Source: CAD feature listing. Evaluate the final solid. Frame: model axes, mm. Face numbers are marked on the shaded views. A direction names the side the tool comes from. Give positions to 0.01 mm unless a question says otherwise; leave off trailing zeros. Order: outer loops, then holes, each group sorted by start corner. A loop starts at its lowest first (then second) coordinate and runs counter-clockwise, first axis right, second up.
1) Section B-B, the plane z = 4.45. Return loops of the section in (x, y), plus the area to 3 significant figures.
2) Draft query along Z for the marked faces 1, 2, 3 and 4. Return one class per face: released by +Z, released by -Z, zero draft, split by the parting line, or undercut.
3) First-contact query: P1, Ø2, axis at y = 4, z = 1, coming from the -X side; P2, Ø1.5, axis at y = 4, z = 4.5, coming from the +X side; P3, Ø0.8, axis at y = 1.5, z = 3, coming from the +X side; P4, Ø0.8, axis at x = -0.5, z = 2.5, coming from the +Y side. Flat tips, straight axial feed; report the tip coordinate or a pass-through.
4) Section C-C, the plane z = 1. Return loops of the section in (x, y), plus the area to 3 significant figures.
5) Section A-A, the plane y = 0.5. Return loops of the section in (x, z).
6) Material intervals for line 1 (Z direction, x = 2, y = 0.3); line 2 (Z direction, x = 0.7, y = 4); line 3 (X direction, y = 1.75, z = 3.9), sorted ascending.
7) Section D-D, the plane x = 2.65. Return loops of the section in (y, z), plus the area to 3 significant figures.
8) Access query for the marked faces 5, 6 and 7. Directions: +Z, -Z, +X, -X, +Y, -Y. A direction counts if a zero-diameter tool reaches every point of the face in a straight line with its end or side. Return the directions, or none.
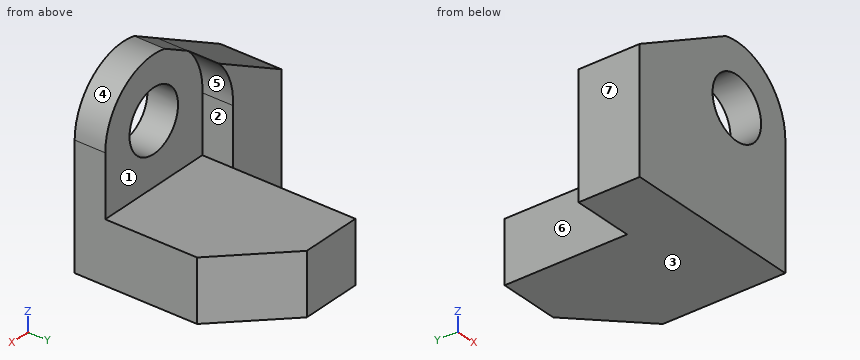
```python
from build123d import *

# Parameters (mm, degrees)
SKETCH1_R           = 1
BOSS_EXTRUDE1_DEPTH = 2
CUT_EXTRUDE1_DEPTH  = 1
SKETCH3_W           = 4
SKETCH3_H           = 2
BOSS_EXTRUDE2_DEPTH = 5
CHAMFER1_SIZE       = 2


with BuildPart() as part:
    # Sketch1 → Boss-Extrude1 (new body)
    with BuildSketch(Plane(origin=(0, 0, 0), x_dir=(1, 0, 0), z_dir=(0, 1, 0))):
        with BuildLine():
            Line((0, -4), (0, 0))
            Line((0, 0), (-2, 0))
            Line((-2, 0), (-2, -4))
            Line((-2, -4), (0.596081752, -5.424434468))
            ThreePointArc((0.596081752, -5.424434468), (0.15502893, -4.772063308), (0, -4))
        make_face()
        with BuildLine():
            Line((4, 0), (0, 0))
            Line((0, 0), (0, -4))
            ThreePointArc((0, -4), (0.15502893, -4.772063308), (0.596081752, -5.424434468))
            Line((0.596081752, -5.424434468), (1.552766589, -5.949354323))
            ThreePointArc((1.552766589, -5.949354323), (3.246100553, -5.56436358), (4, -4))
            Line((4, -4), (4, 0))
        make_face()
        with Locations((2, -4)):
            Circle(SKETCH1_R, mode=Mode.SUBTRACT)
    extrude(amount=BOSS_EXTRUDE1_DEPTH)

    # Sketch2 → Cut-Extrude1 (cut)
    with BuildSketch(Plane(origin=(0, 2, 0), x_dir=(1, 0, 0), z_dir=(0, 1, 0))):
        with BuildLine():
            Line((0, 0), (4, 0))
            Line((4, 0), (4, -4))
            ThreePointArc((4, -4), (1.935634166, -6.000972869), (0, -3.875221449))
            Line((0, -3.875221449), (0, 0))
        make_face()
    extrude(amount=-CUT_EXTRUDE1_DEPTH, mode=Mode.SUBTRACT)

    # Sketch3 → Boss-Extrude2 (add)
    with BuildSketch(Plane(origin=(0, 1, 0), x_dir=(1, 0, 0), z_dir=(0, 1, 0))):
        with Locations((2, -1)):
            Rectangle(SKETCH3_W, SKETCH3_H)
    extrude(amount=BOSS_EXTRUDE2_DEPTH)

    # Chamfer1
    chamfer1_edges = [part.edges().sort_by_distance(p)[0] for p in [
        (4, 6, 1),
    ]]
    chamfer(chamfer1_edges, length=CHAMFER1_SIZE)


solid = part.part
```
From the geometry:
1. outline: (-1.18, 0) - (1.11, 0) - (1.11, 1) - (0.05, 1) - (0.05, 2) - (-1.18, 2) - close; (2.89, 0) - (3.95, 0) - (3.95, 1) - (2.89, 1) - close
1. area: 4.57 mm2
2. face 1: undercut
2. face 2: undercut
2. face 3: released by -Z
2. face 4: released by +Z
3. P1: stops at x = 0
3. P2: passes through
3. P3: stops at x = 0
3. P4: stops at y = 2
4. outline: (-2, 0) - (4, 0) - (4, 4) - (2, 6) - (0, 6) - (0, 2) - (-2, 2) - close
4. area: 26.0 mm2
5. outline: (-2, 0) - (4, 0) - (4, 4) arc R2 ccw to (1.55, 5.95) - (-2, 4) - close; hole circle Ø2 at (2, 4)
6. line 1: z = 0 to 3, 5 to 6
6. line 2: z = 0 to 2
6. line 3: x = -2 to 0
7. outline: (0, 0) - (5.35, 0) - (5.35, 2) - (1, 2) - (1, 3.24) - (0, 3.24) - close; (0, 4.76) - (1, 4.76) - (1, 5.89) - (0, 5.89) - close
7. area: 13.1 mm2
8. face 5: +X, +Y
8. face 6: +Z, -Z, -X, +Y
8. face 7: +Z, -Z, -X, +Y, -Y
